Geometry: final body of the model. Coordinates: model frame, mm. Face numbers are marked on the shaded views. Give positions to 0.01 mm unless a question says otherwise; leave off trailing zeros. Loops run counter-clockwise (first coordinate to the right, second up) from the corner with the lowest first, then second, coordinate; pieces in that order, holes last.
1. Draft query along X for the marked faces 1, 2 and 3. Return one class per face: +X half, -X half, draft (parallel to the pull), parting line (faces both ways), or undercut.
2. Section A-A, the plane x = 0. Output: boundary loops of the cut face in (y, z), then the cut area to 3 significant figures.
3. Section D-D, the plane y = -11.75. Output: boundary loops of the cut face in (x, z), then the cut area to 3 significant figures.
4. Material intervals for line 1 along Y through (x, z) = (0, 3.1); line 2 along Y through (x, z) = (-4.25, 2.65); line 3 along X through (y, z) = (-9.5, 1.55), sorted ascending.
5. First-contact query: P1, Ø3, axis at x = -3.5, y = -4.5, coming from the -Z side. Flat tip, straight axial feed; report the tip coordinate or a pass-through.
6. Section C-C, the plane x = -2.75. Output: boundary loops of the cut face in (y, z), then the cut area to 3 significant figures.
7. Section B-B, the plane z = 1.8. Output: boundary loops of the cut face in (x, y).
from build123d import *

# Parameters (mm, degrees)
CUT_EXTRUDE1_DEPTH      = 16.539441625
CUT_EXTRUDE1_DEPTH_BACK = 16.539441625
SKETCH2_R               = 5


with BuildPart() as part:
    # Sketch1 → Loft1 section 0
    with BuildSketch(Plane.XY):
        with BuildLine():
            Line((6.993136448, 0), (-6.993136448, 0))
            Line((-6.993136448, 0), (-6.993136448, -6.29483871))
            ThreePointArc((-6.993136448, -6.29483871), (0, -13.287975158), (6.993136448, -6.29483871))
            Line((6.993136448, -6.29483871), (6.993136448, 0))
        make_face()
    # Sketch3 → Loft1 section 1
    with BuildSketch(Plane(origin=(0, 0, 4), x_dir=(-1, 0, 0), z_dir=(0, 0, -1))):
        with BuildLine():
            Line((6.993136448, 0), (-6.993136448, 0))
            Line((-6.993136448, 0), (-6.993136448, -6.29483871))
            ThreePointArc((-6.993136448, -6.29483871), (0, -13.287975158), (6.993136448, -6.29483871))
            Line((6.993136448, -6.29483871), (6.993136448, 0))
        make_face()
    loft()

    # Sketch2 → Cut-Extrude1 (cut, two sides: drawn at the far end of the back side and taken through both)
    with BuildSketch(Plane.XY.offset(-CUT_EXTRUDE1_DEPTH_BACK)):
        with Locations((0, -6.29483871)):
            Circle(SKETCH2_R)
    extrude(amount=CUT_EXTRUDE1_DEPTH + CUT_EXTRUDE1_DEPTH_BACK, mode=Mode.SUBTRACT)


solid = part.part
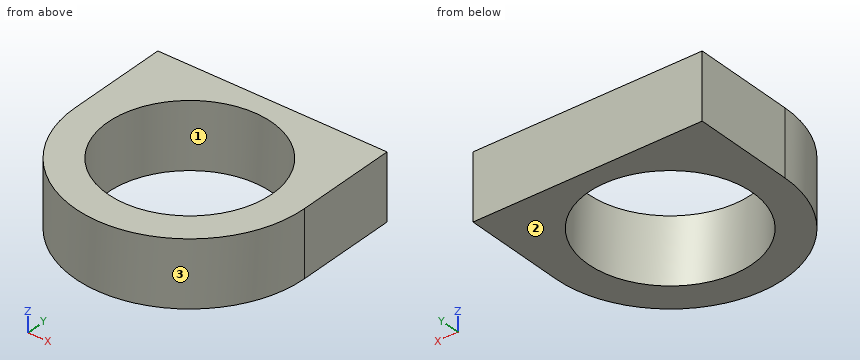
Answers below:
1. face 1: undercut
1. face 2: draft
1. face 3: parting line
2. outline: (-13.29, 0) - (-11.29, 0) - (-11.29, 4) - (-13.29, 4) - close; (-1.29, 0) - (0, 0) - (0, 4) - (-1.29, 4) - close
2. area: 13.2 mm2
3. outline: (-4.38, 0) - (4.38, 0) - (4.38, 4) - (-4.38, 4) - close
3. area: 35.0 mm2
4. line 1: y = -13.29 to -11.29, -1.29 to 0
4. line 2: y = -11.85 to -8.93, -3.66 to 0
4. line 3: x = -6.22 to -3.84, 3.84 to 6.22
5. P1: stops at z = 0
6. outline: (-12.72, 0) - (-10.47, 0) - (-10.47, 4) - (-12.72, 4) - close; (-2.12, 0) - (0, 0) - (0, 4) - (-2.12, 4) - close
6. area: 17.5 mm2
7. outline: (-6.99, -6.29) arc R6.99 ccw to (6.99, -6.29) - (6.99, 0) - (-6.99, 0) - close; hole circle Ø10 at (0, -6.29)
